from build123d import *

# Parameters (mm, degrees)
EXTRUDE_1_DEPTH       = 16
SKETCH_3_R            = 10.75
SKETCH_3_R_2          = 10
EXTRUDE_3_DEPTH       = 294
EXTRUDE_4_DEPTH       = 16
F_1_8_RC_1_AT_2_COUNT = 2
F_1_8_RC_1_AT_2_PITCH = 310
SKETCH_8_R            = 11
EXTRUDE_5_DEPTH       = 12
SKETCH_9_R            = 4
CUT_EXTRUDE_1_DEPTH   = 50
EXTRUDE_START         = 21
SKETCH_10_R           = 11
EXTRUDE_6_DEPTH       = 21
SKETCH_11_R           = 22.5
SKETCH_11_W           = 16
SKETCH_11_H           = 30
CUT_EXTRUDE_2_DEPTH   = 21
SKETCH_12_R           = 4
CUT_EXTRUDE_3_DEPTH   = 339.980733332


with BuildPart() as part:
    # 草图1 → 凸台-拉伸1 (new body)
    with BuildSketch(Plane.XY):
        Polygon((14.5, 0), (7.25, 12.557368355), (-7.25, 12.557368355), (-14.5, 0), (-7.25, -12.557368355), (7.25, -12.557368355), align=None)
    extrude(amount=EXTRUDE_1_DEPTH)

    # 草图3 → 凸台-拉伸3 (add)
    with BuildSketch(Plane.XY.offset(16)):
        Circle(SKETCH_3_R)
        Circle(SKETCH_3_R_2, mode=Mode.SUBTRACT)
    extrude(amount=EXTRUDE_3_DEPTH)

    # 草图4 → 凸台-拉伸4 (add)
    with BuildSketch(Plane.XY.offset(310)):
        Polygon((14.5, 0), (7.25, 12.557368355), (-7.25, 12.557368355), (-14.5, 0), (-7.25, -12.557368355), (7.25, -12.557368355), align=None)
    extrude(amount=EXTRUDE_4_DEPTH)

    # 草图6 → 1/8 Rc 螺纹孔1 (revolve, cut)
    with BuildSketch(Plane(origin=(0, 12.557368355, 318), x_dir=(0, 0, 1), z_dir=(1, 0, 0))):
        Polygon((0, 0), (0, 17.849443543), (3.95, 14.535), (3.95, 10), (3.051996789, 10), (3.364163, 0), align=None)
    f_1_8_rc_1 = revolve(axis=Axis((0, 18.907368355, 318), (0, -1, 0)), mode=Mode.SUBTRACT)

    # 1/8 Rc 螺纹孔1 at 2: 1/8 Rc 螺纹孔1 ×2
    with Locations(*[(0, 0, -i * F_1_8_RC_1_AT_2_PITCH) for i in range(1, F_1_8_RC_1_AT_2_COUNT)]):
        add(f_1_8_rc_1, mode=Mode.SUBTRACT)

    # 草图8 → 凸台-拉伸5 (add)
    with BuildSketch(Plane.XY.offset(326)):
        Circle(SKETCH_8_R)
    extrude(amount=EXTRUDE_5_DEPTH)

    # 草图9 → 切除-拉伸1 (cut)
    with BuildSketch(Plane.XY.offset(338)):
        Circle(SKETCH_9_R)
    extrude(amount=-CUT_EXTRUDE_1_DEPTH, mode=Mode.SUBTRACT)

    # 草图10 → 凸台-拉伸6 (add)
    with BuildSketch(Plane(origin=(0, 0, 0), x_dir=(-1, 0, 0), z_dir=(0, 0, -1)).offset(EXTRUDE_START)):
        with Locations(Location((0, 0, 0), (0, 0, 180))):
            Circle(SKETCH_10_R)
    extrude(amount=-EXTRUDE_6_DEPTH)

    # 草图11 → 切除-拉伸2 (cut)
    with BuildSketch(Plane(origin=(0, 0, -21), x_dir=(-1, 0, 0), z_dir=(0, 0, -1))):
        Circle(SKETCH_11_R)
        Rectangle(SKETCH_11_W, SKETCH_11_H, mode=Mode.SUBTRACT)
    extrude(amount=-CUT_EXTRUDE_2_DEPTH, mode=Mode.SUBTRACT)

    # 草图12 → 切除-拉伸3 (cut, through all)
    with BuildSketch(Plane.ZY.offset(8)):
        with Locations(Location((-9, 0, 0), (0, 0, 270))):
            Circle(SKETCH_12_R)
    extrude(amount=-CUT_EXTRUDE_3_DEPTH, mode=Mode.SUBTRACT)


solid = part.part
Can you work these out from the model? Positions are in its coordinate system, mm. A direction names the side the tool comes from. Round coordinates to 2 decimals unless told otherwise and drop trailing zeros. Write each loop counter-clockwise with the first axis right and the second up, starting at its lowest first coordinate (ties: lowest second). Pieces come first, ordered by that corner, then holes. Notation, with made-up numbers: (-0.5, -17.5) -> (36.5, -17.5) arc R25 cw to (36.5, 5.5) -> close; hole circle Ø7 at (6, -10). An arc over 180 degrees is marked (long way). Use one line per item in the form item = value. Start each with the question number.
Q1. We'd pull the mould along Z, two halves only. Please class faces 5 (the face through (9, 1, 0)), 6 (the face through (-0.112, 0.867, -12.905)), 7 (the face through (-0.141, 7.627, 4.793)), 8 (the face through (10.82, -6.37, 7.89)): +Z half, -Z half, draft (parallel to the pull), parting line (faces both ways), or undercut.
Q2. Imagine slicing it at B-B (z = 92). Please give me the cut outline in (x, y).
Q3. Imagine slicing it at A-A (z = -9). Please give me the cut outline in (x, y), then the cut area to 3 significant figures.
Q4. If I drill on probe 1 along Z at (x, y) = (5, 0); probe 2 along Z at (x, y) = (0, -0.5); probe 3 along Z at (x, y) = (-2, -6), over which ranges is the centre line in solid material (lowest first)? Write a range as [from, to].
Q5. I'm going to push flat-ended pins straight in: P1, Ø5, axis at x = 0, y = 0, coming from the +Z side; P2, Ø1, axis at x = -11.5, z = 199.5, coming from the +Y side; P3, Ø9, axis at y = 0, z = -9, coming from the -X side; P4, Ø1, axis at x = 0, z = 90, coming from the -Y side. Where does each tip first touch, or does it pass through?
Q6. Which directions (+Z, -Z, +X, -X, +Y, -Y) give clear straight access to the entire face, cutting with the end or side of a thin tool? Please do faces 1 (the face through (-8, 2, -13)), 2 (the face through (8, 2, -13)), 3 (the face through (3, 2.557, 10)), 4 (the face through (-4, 0, 324)).
Worked out:
q1.face_5 = -Z half
q1.face_6 = undercut
q1.face_7 = undercut
q1.face_8 = draft
q2.outline = circle Ø21.5 at (0, 0); hole circle Ø20 at (0, 0)
q3.outline = (-8, -7.55) arc R11 ccw to (8, -7.55) -> (8, -4) -> (-8, -4) -> close; (-8, 4) -> (8, 4) -> (8, 7.55) arc R11 ccw to (-8, 7.55) -> close
q3.area = 190 mm^2
q4.probe_1 = [-21, -13], [-5, 16], [310, 338]
q4.probe_2 = [-21, -12.97], [-5.03, 4.05], [11.95, 16]
q4.probe_3 = [-21, 16], [310, 338]
q5.P1 = 16
q5.P2 = through
q5.P3 = -8
q5.P4 = -10.75
q6.face_1 = -Z, -X, +Y, -Y
q6.face_2 = -Z, +X, +Y, -Y
q6.face_3 = none
q6.face_4 = +Z
